Input: part model. Units: mm. Frame: model coordinates. A direction names the side the tool comes from. Coordinates: 2 decimals unless noted, no trailing zeros. Loops run counter-clockwise (first coordinate to the right, second up) from the corner with the lowest first, then second, coordinate; pieces in that order, holes last. Notation, with made-up numbers: (-3, 79.5) - (27, 79.5) arc R22 ccw to (27, 114.5) - close; hole circle Ø8 at (21, -9.5). An arc over 180 degrees is marked (long way). Use a Markdown table: item, result. Add a question column.
1. Access query for faces 4 (the face through (-40.995, 12.722, 1.39)), 5 (the face through (-35, 41, 38.1)). Directions: +Z, -Z, +X, -X, +Y, -Y. A direction counts if a zero-diameter tool reaches every point of the face in a straight line with its end or side. Return the directions, or none.
2. Ray query, L1, parallel to X at y = 8.5, z = 2. Return the intervals inside material, ascending. Write a range as [from, to].
3. Contact query for a flat-ended pin moving along its axis: P1, Ø4, axis at x = -42, y = 8, coming from the -Z side. Output: stop coordinate, or through.
4. Draft query along X for faces 1 (the face through (-41, 5, 2.819)), 2 (the face through (-69.85, 41, 19)), 3 (the face through (-35, 41, 0)). Return one class per face: released by +X, released by -X, zero draft, split by the parting line, or undercut.
5. Section query A-A on y = 10. Return the cut outline in (x, z), then the cut area to 3 significant figures.
```python
from build123d import *

# Parameters (mm, degrees)
SKETCH1_W           = 82.55
SKETCH1_H           = 69.85
BOSS_EXTRUDE1_DEPTH = 38.1
SKETCH2_R           = 12.7254
CUT_EXTRUDE1_DEPTH  = 2.8194


with BuildPart() as part:
    # Sketch1 → Boss-Extrude1 (new body)
    with BuildSketch(Plane(origin=(0, 0, 0), x_dir=(0, 1, 0), z_dir=(0, 0, 1))):
        with Locations((41.275, 34.925)):
            Rectangle(SKETCH1_W, SKETCH1_H)
    extrude(amount=BOSS_EXTRUDE1_DEPTH)

    # Sketch2 → Cut-Extrude1 (cut)
    with BuildSketch(Plane(origin=(0, 0, 0), x_dir=(0, 1, 0), z_dir=(0, 0, 1))):
        with Locations((0, 41.275)):
            Circle(SKETCH2_R)
    extrude(amount=CUT_EXTRUDE1_DEPTH, mode=Mode.SUBTRACT)


solid = part.part
```
Resolved:
| question | item | result |
|---|---|---|
| 1 | face 4 | -Z, -Y |
| 1 | face 5 | +Z, +X, -X, +Y, -Y |
| 2 | L1 | [-69.85, -50.75], [-31.8, 0] |
| 3 | P1 | z = 2.82 |
| 4 | face 1 | undercut |
| 4 | face 2 | released by -X |
| 4 | face 3 | zero draft |
| 5 | outline | (-69.85, 0) - (-49.14, 0) - (-49.14, 2.82) - (-33.41, 2.82) - (-33.41, 0) - (0, 0) - (0, 38.1) - (-69.85, 38.1) - close |
| 5 | area | 2,620 mm² |
